Could you check a few things on this drawing? It's one solid part, dimensions in mm from its lowest x, y, z. Give positions to 0.01 mm unless a question says otherwise; leave off trailing zeros. Loops run counter-clockwise (first coordinate to the right, second up) from the corner with the lowest first, then second, coordinate; pieces in that order, holes last. Notation, with made-up numbers: (-24, -27.75) - (24, -27.75) arc R12 ccw to (24, -10.75) - close; hole circle Ø7 at (-12.75, 37). An arc over 180 degrees is marked (long way). Return JSON: item names as keys, results as strings. Group by question number.
(1) If we section it at B-B (y = 101): Please give me the cut outline in (x, z).
(2) If we section it at C-C (z = 1.75): State how many separate pieces and enclosed holes the cut face has, then the cut area to 3 significant figures.
(3) If we section it at D-D (y = 117): Please give me the cut outline in (x, z).
(4) I need wall thicknesses on probe 1 along X at (y, z) = (64.5, 3.25) (1 decimal); probe 2 along Y at (x, z) = (184.15, 4.25); probe 3 along Y at (x, z) = (108, 3.75). Which ranges of each line are inside material? Lowest first, please. Write a range as [from, to].
(5) For P1, Ø2, axis at x = 23, z = 3, coming from the +Y side; P2, Ø2, axis at y = 44, z = 3.5, coming from the -X side, each with a flat end and sliding along its axis, tell me the tip position at first contact or that it passes through.
(6) If we section it at A-A (x = 107.95): Please give me the cut outline in (y, z).
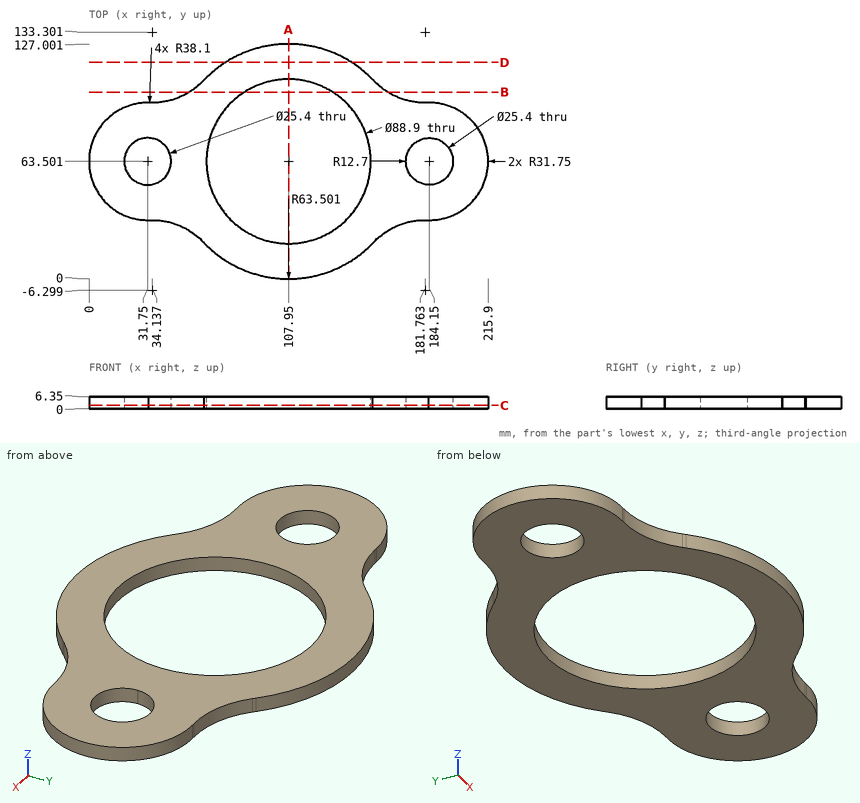
Values:
{
 "1": {"outline": "(54.34, 0) - (84.08, 0) - (84.08, 6.35) - (54.34, 6.35) - close; (131.82, 0) - (161.56, 0) - (161.56, 6.35) - (131.82, 6.35) - close"},
 "2": {"separate pieces": "1", "enclosed holes": "3", "area": "10,800 mm2"},
 "3": {"outline": "(73.74, 0) - (142.16, 0) - (142.16, 6.35) - (73.74, 6.35) - close"},
 "4": {"probe 1": "[0, 19.1], [44.4, 63.5], [152.4, 171.5], [196.8, 215.9]", "probe 2": "[31.75, 50.8], [76.2, 95.25]", "probe 3": "[0, 19.05], [107.95, 127]"},
 "5": {"P1": "y = 94.29", "P2": "x = 5.95"},
 "6": {"outline": "(0, 0) - (19.05, 0) - (19.05, 6.35) - (0, 6.35) - close; (107.95, 0) - (127, 0) - (127, 6.35) - (107.95, 6.35) - close"}
}
